```python
from build123d import *

# Parameters (mm, degrees)
F0_R     = 32.25
F1_DEPTH = 155
F2_R     = 20.142482
F3_DEPTH = 30
F4_R     = 10
F5_R     = 6
F6_DEPTH = 16
F7_R     = 2


with BuildPart() as f1:
    # F0 (on Top) → F1 (new body)
    with BuildSketch(Plane.XY):
        Circle(F0_R)
    extrude(amount=F1_DEPTH)

    # F2 (on face) → F3 (join)
    with BuildSketch(Plane.XY.offset(155)):
        Circle(F2_R)
    extrude(amount=F3_DEPTH)

    # F4
    f4_edges = [f1.edges().sort_by_distance(p)[0] for p in [
        (-20.142482, 0, 185),
    ]]
    fillet(f4_edges, radius=F4_R)

    # F5 (on face) → F6 (join)
    with BuildSketch(Plane(origin=(0, 0, 0), x_dir=(1, 0, 0), z_dir=(0, 0, -1))):
        Circle(F5_R)
    extrude(amount=F6_DEPTH)

    # F7
    f7_edges = [f1.edges().sort_by_distance(p)[0] for p in [
        (-32.25, 0, 155),
        (-32.25, 0, 0),
    ]]
    fillet(f7_edges, radius=F7_R)


solid = f1.part
```
Input: part model. Units: mm. Frame: model coordinates. A direction names the side the tool comes from. Give positions to 0.01 mm unless a question says otherwise; leave off trailing zeros. Write each loop counter-clockwise with the first axis right and the second up, starting at its lowest first coordinate (ties: lowest second). Pieces come first, ordered by that corner, then holes. Notation, with made-up numbers: (17, -14.5) - (24, -14.5) arc R24 cw to (24, 7.5) - close; hole circle Ø4 at (35, -34.5). An arc over 180 degrees is marked (long way). Write item = value, one per line. Start each with the question number.
1) Cut plane A-A (y = 0). Return loops of the section in (x, z).
2) Reachability of faces 1 (the face through (0, 0, 185)), 2 (the face through (20, -6, 155)), 3 (the face through (-6, 0, -8)) from +Z, -Z, +X, -X, +Y, -Y: full face, straight path, thin tool, end or side. Return the list, or none.
3) Pin query (flat end, axial travel): pin 1 (1.5 mm diameter, centred on x = -10.5, y = -24, fed in from -Z); pin 2 (1.5 mm diameter, centred on y = -3.5, z = 115.5, fed in from -X); pin 3 (4 mm diameter, centred on y = 13.5, z = 140, fed in from +X). Return the tip coordinate at first contact, or that it passes through.
4) Material intervals for L1, parallel to Z at x = 1, y = -9.5; L2, parallel to Z at x = 20, y = -18.5; L3, parallel to Y at x = 0, z = 3, sorted ascending. Write a range as [from, to].
5) Cut plane C-C (z = 39.5). Return loops of the section in (x, y).
Answers follow:
q1.outline = (-32.25, 2) arc R2 ccw to (-30.25, 0) - (-6, 0) - (-6, -16) - (6, -16) - (6, 0) - (30.25, 0) arc R2 ccw to (32.25, 2) - (32.25, 153) arc R2 ccw to (30.25, 155) - (20.14, 155) - (20.14, 175) arc R10 ccw to (10.14, 185) - (-10.14, 185) arc R10 ccw to (-20.14, 175) - (-20.14, 155) - (-30.25, 155) arc R2 ccw to (-32.25, 153) - close
q2.face_1 = +Z, +X, -X, +Y, -Y
q2.face_2 = +Z
q2.face_3 = -Z
q3.pin_1 = 0
q3.pin_2 = -32.13
q3.pin_3 = 30.13
q4.L1 = [0, 185]
q4.L2 = [0, 155]
q4.L3 = [-32.25, 32.25]
q5.outline = circle Ø64.5 at (0, 0)
